Geometry: final body of the model. Coordinates: model frame, mm. A direction names the side the tool comes from. Round coordinates to 2 decimals unless told otherwise and drop trailing zeros. Write each loop counter-clockwise with the first axis right and the second up, starting at its lowest first coordinate (ties: lowest second). Pieces come first, ordered by that corner, then holes. Notation, with made-up numbers: M -25,-22 L 25,-22 A16 cw 25,-3 Z; hole C 52.5,33 d1. An arc over 180 degrees is marked long. Use one line per item in the form item = value. Start each with the question number.
from build123d import *

# Parameters (mm, degrees)
F0_R      = 37.5
F0_R_2    = 35
F1_DEPTH  = 25
F2_R      = 42.5
F2_R_2    = 35
F3_DEPTH  = 10
F4_R      = 5
F6_R      = 37.5
F6_R_2    = 36.5
F7_DEPTH  = 5
F9_DEPTH  = 3
F11_DEPTH = 3


with BuildPart() as f1:
    # F0 (on Front) → F1 (new body)
    with BuildSketch(Plane.XZ):
        Circle(F0_R)
        Circle(F0_R_2, mode=Mode.SUBTRACT)
    extrude(amount=F1_DEPTH)

    # F2 (on face) → F3 (join)
    with BuildSketch(Plane.XZ.offset(25)):
        Circle(F2_R)
        Circle(F2_R_2, mode=Mode.SUBTRACT)
    extrude(amount=F3_DEPTH)

    # F4
    f4_edges = [f1.edges().sort_by_distance(p)[0] for p in [
        (-35, -35, 0),
    ]]
    fillet(f4_edges, radius=F4_R)

    # F6 (on offset) → F7 (cut)
    with BuildSketch(Plane.XZ.offset(5)):
        Circle(F6_R)
        Circle(F6_R_2, mode=Mode.SUBTRACT)
    extrude(amount=F7_DEPTH, mode=Mode.SUBTRACT)

    # F8 (on offset) → F9 (join)
    with BuildSketch(Plane.XZ.offset(5)):
        with BuildLine():
            Line((27.399526, 9.749617), (33.614654, 9.749617))
            ThreePointArc((33.614654, 9.749617), (0.227268, 34.999262), (-33.485206, 10.185331))
            Line((-33.485206, 10.185331), (-27.24056, 10.185331))
            ThreePointArc((-27.24056, 10.185331), (0.231904, 29.081528), (27.399526, 9.749617))
        make_face()
    extrude(amount=F9_DEPTH)

    # F10 (on offset) → F11 (join)
    with BuildSketch(Plane.XZ.offset(5)):
        with BuildLine():
            Line((-28.114079, -7.974047), (-34.079533, -7.974047))
            ThreePointArc((-34.079533, -7.974047), (-0.106236, -34.999839), (34.030498, -8.180783))
            Line((34.030498, -8.180783), (28.054619, -8.180783))
            ThreePointArc((28.054619, -8.180783), (-0.107558, -29.222855), (-28.114079, -7.974047))
        make_face()
    extrude(amount=F11_DEPTH)


solid = f1.part
1. Pull-direction query (Y, two-part tool) for faces 1 (the face through (-31, 0, 17)), 2 (the face through (8, -10, -36)), 3 (the face through (0.42, -6.48, -29.22)); classes: released by +Y, released by -Y, zero draft, split by the parting line, or undercut.
2. Section query C-C (y = -14.5). Return loops of the section in (x, z), then the cut area to 3 significant figures.
3. Section query D-D (y = -32). Return loops of the section in (x, z), then the cut area to 3 significant figures.
4. Set-up query: faces 4 (the face through (31, -6, -8.181)), 5 (the face through (0, -25, -38)), 6 (the face through (-0.2, -8, -29.4)), 7 (the face through (-28, -15, -21)). Return all of +Z, -Z, +X, -X, +Y, -Y with unobstructed straight access to the full face (end or side cutting, diameter ignored); none if empty.
5. Contact query for flat-ended pins moving along their axis: pin 1 (6 mm diameter, centred on y = -6.5, z = -9, fed in from -X); pin 2 (10 mm diameter, centred on y = -18.5, z = 11, fed in from +X); pin 3 (6 mm diameter, centred on x = 12, z = 29, fed in from +Y); pin 4 (12 mm diameter, centred on x = 12.5, z = -12.5, fed in from -Y). Output: stop coordinate, or through.
6. Ray query, probe 1 along Z at (x, y) = (0, -14); probe 2 along Z at (x, y) = (0, -9); probe 3 along X at (y, z) = (-27, -0.5). Return the intervals inside material, ascending.
7. Section query A-A (z = 0). Return loops of the section in (x, y).
Checks:
q1.face_1 = released by +Y
q1.face_2 = undercut
q1.face_3 = zero draft
q2.outline = C 0,0 d75; hole C 0,0 d70
q2.area = 569 mm^2
q3.outline = C 0,0 d85; hole C 0,0 d70.83
q3.area = 1,730 mm^2
q4.face_4 = +Y, -Y
q4.face_5 = +Y
q4.face_6 = -Y
q4.face_7 = none
q5.pin_1 = -36.95
q5.pin_2 = 37.02
q5.pin_3 = -5
q5.pin_4 = through
q6.probe_1 = -37.5 to -35, 35 to 37.5
q6.probe_2 = -36.5 to -35, 35 to 36.5
q6.probe_3 = -42.5 to -35, 35 to 42.5
q7.outline = M -42.5,-35 L -40,-35 A5 ccw -35,-30 L -35,0 L -37.5,0 L -37.5,-5 L -36.5,-5 L -36.5,-10 L -37.5,-10 L -37.5,-25 L -42.5,-25 Z; M 35,-30 A5 ccw 40,-35 L 42.5,-35 L 42.5,-25 L 37.5,-25 L 37.5,-10 L 36.5,-10 L 36.5,-5 L 37.5,-5 L 37.5,0 L 35,0 Z
